Could you check a few things on this model? Use its own coordinates, in mm. Give positions to 0.01 mm unless a question says otherwise; leave off trailing zeros. Loops run counter-clockwise (first coordinate to the right, second up) from the corner with the lowest first, then second, coordinate; pieces in that order, holes last. Notation, with made-up numbers: M 42.25,39 L 92.25,39 A17 ccw 92.25,71 Z; hole C 5.5,23 d9. An arc over 180 degrees is marked long. Answer in a Markdown table with one row per item. Add a question column.
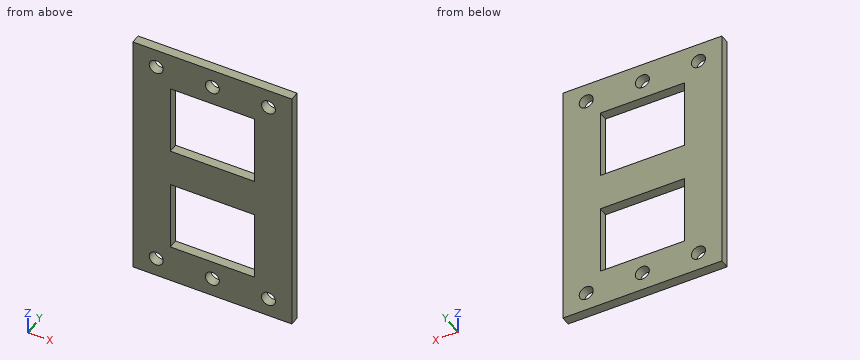
Autodesk Inventor part; units mm, degrees
ref_plane "YZ Plane" through (0, 0, 0) normal (1, 0, 0) x (0, 1, 0)
ref_plane "XZ Plane" through (0, 0, 0) normal (0, 1, 0) x (-1, 0, 0)
ref_plane "XY Plane" through (0, 0, 0) normal (0, 0, 1) x (1, 0, 0)
sketch "Sketch1" plane through (0, 0, 0) normal (0, 1, 0) x (-1, 0, 0)
  line L0 (169.9997, 270) -> (-169.9997, 270)
  line L1 (-169.9997, 270) -> (-169.9997, -270)
  line L2 (-169.9997, -270) -> (169.9997, -270)
  line L3 (169.9997, -270) -> (169.9997, 270)
  line L4 (169.9997, 270) -> (-169.9997, -270) construction
  line L5 (-169.9997, 270) -> (169.9997, -270) construction
  point P0 (0, 0)
  dimension "d0" = 339.9993
  dimension "d1" = 539.9999
extrude "Extrusion1" add sketch "Sketch1" along normal blind 20.0025
sketch "Sketch2" plane through (0, 20.0025, 0) normal (0, 1, 0) x (1, 0, 0)
  line L0 (-89.916, 189.8523) -> (89.916, 189.8523)
  line L1 (89.916, 189.8523) -> (89.916, 39.9923)
  line L2 (89.916, 39.9923) -> (-89.916, 39.9923)
  line L3 (-89.916, 39.9923) -> (-89.916, 189.8523)
  line L4 (-89.916, 189.8523) -> (89.916, 39.9923) construction
  line L5 (89.916, 189.8523) -> (-89.916, 39.9923) construction
  line L6 (-89.916, -39.9923) -> (89.916, -39.9923)
  line L7 (89.916, -39.9923) -> (89.916, -189.8523)
  line L8 (89.916, -189.8523) -> (-89.916, -189.8523)
  line L9 (-89.916, -189.8523) -> (-89.916, -39.9923)
  line L10 (-89.916, -39.9923) -> (89.916, -189.8523) construction
  line L11 (89.916, -39.9923) -> (-89.916, -189.8523) construction
  line L12 (-169.9997, -270) -> (169.9997, -270)
  line L13 (0, 0) -> (-323.2387, 0) construction
  point P0 (0, 114.9223)
  point P1 (0, -114.9223)
  point P2 (0, -114.9223)
  dimension "d4" = 149.86
  dimension "d5" = 149.86
  dimension "d6" = 179.832
  dimension "d7" = 179.832
  dimension "d9" = 79.9846
extrude "Extrusion2" cut sketch "Sketch2" against normal through all
hole "Hole1" at (-119.9998, 20.0025, 229.995) direction (0, -1, 0) diameter 29.9999 end through all
pattern_linear "Rectangular Pattern1" count 2 spacing 459.994 along (0, 0, -1) count 3 spacing 119.9998 along (1, 0, 0) of "Hole1"
Item 1: Suppose I cut it at D-D (z = -225.5). List the corners of the cut face in (x, y) for me, then the cut area to 3 significant figures.
Item 2: Suppose I cut it at A-A (x = -53.5). List the corners of the cut face in (y, z) for me, then the cut area to 3 significant figures.
Item 3: For P1, Ø24, axis at x = 120, z = -230, coming from the -Y side, with a flat end and sliding along its axis, tell me the tip position at first contact or that it passes through.
Item 4: Suppose I cut it at B-B (z = 72). List the corners of the cut face in (x, y) for me.
Item 5: Suppose I cut it at C-C (x = 0). List the corners of the cut face in (y, z) for me, then the cut area to 3 significant figures.
Item 6: I need wall thicknesses on L1, parallel to Z at x = 0, y = 10; L2, parallel to X at y = 6.5, z = 168; L3, parallel to Z at x = 49, y = 16.5. Which ranges of each line are inside material? Lowest first, please.
Values found:
| question | item | result |
|---|---|---|
| 1 | outline | M -170,0 L -134.31,0 L -134.31,20 L -170,20 Z; M -105.69,0 L -14.31,0 L -14.31,20 L -105.69,20 Z; M 14.31,0 L 105.69,0 L 105.69,20 L 14.31,20 Z; M 134.31,0 L 170,0 L 170,20 L 134.31,20 Z |
| 1 | area | 5,080 mm² |
| 2 | outline | M 0,-270 L 20,-270 L 20,-189.85 L 0,-189.85 Z; M 0,-39.99 L 20,-39.99 L 20,39.99 L 0,39.99 Z; M 0,189.85 L 20,189.85 L 20,270 L 0,270 Z |
| 2 | area | 4,810 mm² |
| 3 | P1 | through |
| 4 | outline | M -170,0 L -89.92,0 L -89.92,20 L -170,20 Z; M 89.92,0 L 170,0 L 170,20 L 89.92,20 Z |
| 5 | outline | M 0,-270 L 20,-270 L 20,-245 L 0,-245 Z; M 0,-215 L 20,-215 L 20,-189.85 L 0,-189.85 Z; M 0,-39.99 L 20,-39.99 L 20,39.99 L 0,39.99 Z; M 0,189.85 L 20,189.85 L 20,215 L 0,215 Z; M 0,244.99 L 20,244.99 L 20,270 L 0,270 Z |
| 5 | area | 3,610 mm² |
| 6 | L1 | -270 to -245, -215 to -189.85, -39.99 to 39.99, 189.85 to 215, 244.99 to 270 |
| 6 | L2 | -170 to -89.92, 89.92 to 170 |
| 6 | L3 | -270 to -189.85, -39.99 to 39.99, 189.85 to 270 |
